Autodesk Inventor part; units mm, degrees
ref_plane "YZ Plane" through (0, 0, 0) normal (1, 0, 0) x (0, 1, 0)
ref_plane "XZ Plane" through (0, 0, 0) normal (0, 1, 0) x (-1, 0, 0)
ref_plane "XY Plane" through (0, 0, 0) normal (0, 0, 1) x (1, 0, 0)
sketch "Sketch1" plane through (0, 0, 0) normal (0, 1, 0) x (-1, 0, 0)
  line L0 (0, 0) -> (101.6, 0)
  line L1 (101.6, 0) -> (101.6, -101.6)
  line L2 (101.6, -101.6) -> (0, -101.6)
  line L3 (0, -101.6) -> (0, 0)
  dimension "d0" = 101.6
  dimension "d1" = 101.6
extrude "Extrusion1" add sketch "Sketch1" along normal blind 6.35 draft 0.25
sketch "Sketch2" plane through (0, 6.35, 0) normal (0, 1, 0) x (1, 0, 0)
  line L0 (-82.5492, 50.8025) -> (-86.8726, 48.5826)
  line L1 (-86.8726, 48.5826) -> (-82.3808, 47.537)
  line L2 (-82.3808, 47.537) -> (-86.5353, 45.4037)
  line L3 (-86.5353, 45.4037) -> (-81.9297, 44.5615)
  line L4 (-81.9297, 44.5615) -> (-85.8551, 42.0104)
  line L5 (-85.8551, 42.0104) -> (-81.2075, 41.6704)
  line L6 (-81.2075, 41.6704) -> (-84.931, 38.9182)
  line L7 (-84.931, 38.9182) -> (-80.2411, 38.9182)
  line L8 (-80.2411, 38.9182) -> (-83.7111, 35.8686)
  line L9 (-83.7111, 35.8686) -> (-78.9909, 36.1982)
  line L10 (-78.9909, 36.1982) -> (-82.2207, 32.9446)
  line L11 (-82.2207, 32.9446) -> (-77.3914, 33.4556)
  line L12 (-77.3914, 33.4556) -> (-80.2618, 29.8701)
  line L13 (-80.2618, 29.8701) -> (-75.5543, 30.9218)
  line L14 (-75.5543, 30.9218) -> (-78.0086, 27.0147)
  line L15 (-78.0086, 27.0147) -> (-73.2491, 28.3512)
  line L16 (-75.4686, 24.3897) -> (-70.7203, 26.0798)
  line L17 (-70.7203, 26.0798) -> (-72.3407, 21.7822)
  line L18 (-72.3407, 21.7822) -> (-67.7356, 23.947)
  line L19 (-67.7356, 23.947) -> (-68.5334, 19.3111)
  line L20 (-68.5334, 19.3111) -> (-64.1946, 22.0167)
  line L21 (-64.1946, 22.0167) -> (-64.3717, 17.3062)
  line L22 (-64.3717, 17.3062) -> (-60.4516, 20.5554)
  line L23 (-60.4516, 20.5554) -> (-60.1774, 15.8989)
  line L24 (-60.1774, 15.8989) -> (-56.5068, 19.5698)
  line L25 (-56.5068, 19.5698) -> (-55.1527, 14.9241)
  line L26 (-55.1527, 14.9241) -> (-52.5263, 19.0996)
  line L27 (-52.5263, 19.0996) -> (-50.7684, 14.6609)
  line L28 (-50.7684, 14.6609) -> (-48.585, 19.1298)
  line L29 (-48.585, 19.1298) -> (-46.5035, 14.9171)
  line L30 (-46.5035, 14.9171) -> (-45.1599, 19.5574)
  line L31 (-45.1599, 19.5574) -> (-42.5914, 15.6053)
  line L32 (-42.5914, 15.6053) -> (-41.7527, 20.3686)
  line L33 (-41.7527, 20.3686) -> (-39.298, 16.5397)
  line L34 (-39.298, 16.5397) -> (-38.6769, 21.4578)
  line L35 (-38.6769, 21.4578) -> (-35.49, 18.0635)
  line L36 (-35.49, 18.0635) -> (-35.1146, 23.1972)
  line L37 (-35.1146, 23.1972) -> (-30.9781, 20.581)
  line L38 (-30.9781, 20.581) -> (-31.5036, 25.5886)
  line L39 (-31.5036, 25.5886) -> (-27.2251, 23.4077)
  line L40 (-27.2251, 23.4077) -> (-28.4283, 28.2724)
  line L41 (-28.4283, 28.2724) -> (-23.9858, 26.5691)
  line L42 (-23.9858, 26.5691) -> (-26.0364, 30.9313)
  line L43 (-26.0364, 30.9313) -> (-21.3587, 29.8388)
  line L44 (-21.3587, 29.8388) -> (-23.7723, 34.1409)
  line L45 (-23.7723, 34.1409) -> (-18.848, 33.9105)
  line L46 (-18.848, 33.9105) -> (-22.0511, 37.3262)
  line L47 (-22.0511, 37.3262) -> (-17.264, 37.3262)
  line L48 (-17.264, 37.3262) -> (-20.7009, 40.6952)
  line L49 (-20.7009, 40.6952) -> (-15.918, 41.3408)
  line L50 (-15.918, 41.3408) -> (-19.7237, 44.293)
  line L51 (-19.7237, 44.293) -> (-15.0837, 45.2689)
  line L52 (-15.0837, 45.2689) -> (-19.1835, 47.8849)
  line L53 (-19.1835, 47.8849) -> (-14.7085, 48.8843)
  line L54 (-14.7085, 48.8843) -> (-19.0492, 50.8025)
  line L55 (-75.4686, 24.3897) -> (-73.2491, 28.3512)
  circle A0 centre (-50.8, 50.8) radius 31.7508
  circle A1 centre (-50.8, 50.8) radius 37.6285
  line L56 (-101.6277, 101.6277) -> (0.0277, 101.6277)
  line L57 (0.0277, 101.6277) -> (0.0277, -0.0277)
  line L58 (-101.6277, 101.6277) -> (0.0277, 101.6277)
  line L59 (0.0277, 101.6277) -> (0.0277, -0.0277)
  line L60 (0.0277, -0.0277) -> (-101.6277, -0.0277)
  line L61 (0.0277, -0.0277) -> (-101.6277, -0.0277)
  line L62 (-101.6277, -0.0277) -> (-101.6277, 101.6277)
extrude "Extrusion2" cut sketch "Sketch2" against normal blind 6.35 contours L56 L57 L60 L62
sketch "Sketch3" plane through (-50.8, 6.35, -50.8) normal (0, 1, 0) x (1, 0, 0)
  line L0 (-31.7492, 0.0025) -> (-36.0726, -2.2174)
  line L1 (-36.0726, -2.2174) -> (-31.5808, -3.263)
  line L2 (-31.5808, -3.263) -> (-35.7353, -5.3963)
  line L3 (-35.7353, -5.3963) -> (-31.1298, -6.2385)
  line L4 (-31.1298, -6.2385) -> (-35.0551, -8.7896)
  line L5 (-35.0551, -8.7896) -> (-30.4075, -9.1296)
  line L6 (-30.4075, -9.1296) -> (-34.131, -11.8818)
  line L7 (-34.131, -11.8818) -> (-29.4411, -11.8818)
  line L8 (-29.4411, -11.8818) -> (-32.9111, -14.9315)
  line L9 (-32.9111, -14.9315) -> (-28.191, -14.6019)
  line L10 (-28.191, -14.6019) -> (-31.4207, -17.8554)
  line L11 (-31.4207, -17.8554) -> (-26.5914, -17.3444)
  line L12 (-26.5914, -17.3444) -> (-29.4619, -20.9299)
  line L13 (-29.4619, -20.9299) -> (-24.7544, -19.8782)
  line L14 (-24.7544, -19.8782) -> (-27.2087, -23.7853)
  line L15 (-27.2087, -23.7853) -> (-22.4492, -22.4488)
  line L16 (-24.6686, -26.4103) -> (-19.9203, -24.7202)
  line L17 (-19.9203, -24.7202) -> (-21.5408, -29.0178)
  line L18 (-21.5408, -29.0178) -> (-16.9357, -26.853)
  line L19 (-16.9357, -26.853) -> (-17.7335, -31.489)
  line L20 (-17.7335, -31.489) -> (-13.3947, -28.7833)
  line L21 (-13.3947, -28.7833) -> (-13.5717, -33.4938)
  line L22 (-13.5717, -33.4938) -> (-9.6516, -30.2447)
  line L23 (-9.6516, -30.2447) -> (-9.3774, -34.9011)
  line L24 (-9.3774, -34.9011) -> (-5.7069, -31.2302)
  line L25 (-5.7069, -31.2302) -> (-4.3528, -35.8759)
  line L26 (-4.3528, -35.8759) -> (-1.7263, -31.7005)
  line L27 (-1.7263, -31.7005) -> (0.0315, -36.1391)
  line L28 (0.0315, -36.1391) -> (2.215, -31.6702)
  line L29 (2.215, -31.6702) -> (4.2964, -35.8829)
  line L30 (4.2964, -35.8829) -> (5.64, -31.2426)
  line L31 (5.64, -31.2426) -> (8.2086, -35.1948)
  line L32 (8.2086, -35.1948) -> (9.0473, -30.4314)
  line L33 (9.0473, -30.4314) -> (11.502, -34.2603)
  line L34 (11.502, -34.2603) -> (12.123, -29.3422)
  line L35 (12.123, -29.3422) -> (15.3099, -32.7365)
  line L36 (15.3099, -32.7365) -> (15.6854, -27.6028)
  line L37 (15.6854, -27.6028) -> (19.8219, -30.219)
  line L38 (19.8219, -30.219) -> (19.2964, -25.2114)
  line L39 (19.2964, -25.2114) -> (23.5749, -27.3924)
  line L40 (23.5749, -27.3924) -> (22.3717, -22.5276)
  line L41 (22.3717, -22.5276) -> (26.8141, -24.2309)
  line L42 (26.8141, -24.2309) -> (24.7636, -19.8687)
  line L43 (24.7636, -19.8687) -> (29.4412, -20.9612)
  line L44 (29.4412, -20.9612) -> (27.0277, -16.6591)
  line L45 (27.0277, -16.6591) -> (31.9519, -16.8895)
  line L46 (31.9519, -16.8895) -> (28.7489, -13.4738)
  line L47 (28.7489, -13.4738) -> (33.5359, -13.4738)
  line L48 (33.5359, -13.4738) -> (30.099, -10.1049)
  line L49 (30.099, -10.1049) -> (34.8819, -9.4592)
  line L50 (34.8819, -9.4592) -> (31.0763, -6.5071)
  line L51 (31.0763, -6.5071) -> (35.7163, -5.5311)
  line L52 (35.7163, -5.5311) -> (31.6164, -2.9151)
  line L53 (31.6164, -2.9151) -> (36.0915, -1.9157)
  line L54 (36.0915, -1.9157) -> (31.7508, 0.0025)
  line L55 (-24.6686, -26.4103) -> (-22.4492, -22.4488)
  line L56 (-31.7492, 0.0025) -> (31.7508, 0.0025)
  circle A0 centre (0.0008, 0.0025) radius 37.6862
  point P0 (50.8, -50.8)
extrude "Extrusion3" cut sketch "Sketch3" against normal blind 6.35
For this review, take the finished solid that the model builds, in its own axes (mm). A direction names the side the tool comes from. Coordinates: 2 decimals unless noted, no trailing zeros. Write each loop counter-clockwise with the first axis right and the second up, starting at its lowest first coordinate (ties: lowest second). Pieces come first, ordered by that corner, then holes.
(1) Tool access review of faces 1 (the face through (-27.82, 3.22, -25.81)), 2 (the face through (-51.66, 3.22, -16.91)), 3 (the face through (-16.85, 3.22, -49.83)), 4 (the face through (-18.343, 3.219, -41.013)): name each direction out of +Z, -Z, +X, -X, +Y, -Y from which nothing blocks a thin tool from reaching the whole face with its end or side.
(2) Wall thickness on probe 1 along X at (y, z) = (0.5, -21); probe 2 along Z at (x, y) = (-80.5, 3.75); probe 3 along Z at (x, y) = (-23.5, 1.5): over which ranges is each line inside the solid? List them lowest first.
(3) The part is to be moulded in two halves that separate along X. For faces 5 (the face through (-81.38, 3.22, -36.03)), 6 (the face through (-17.8, 3.2, -42.8)), 7 (the face through (-58.368, 3.219, -17.709)), say which applies: +X half, -X half, draft (parallel to the pull), parting line (faces both ways), or undercut.
(4) For pin 1 Ø1 at (y, z) = (4.5, -24) entering from -X; pin 2 Ø1 at (y, z) = (1, -25) entering from +X; pin 3 Ø1 at (y, z) = (0.5, -29) entering from +X, all flat-tipped, find the tip position at first contact; note any pin that passes through.
(5) Add section B-B on x = -43.5. Give the boundary of the cut face in (y, z), then the cut area to 3 significant figures.
(6) Add section C-C on z = -43.5. Give the boundary of the cut face in (x, y), then the cut area to 3 significant figures.
(7) Add section A-A on x = -74. Give the boundary of the cut face in (y, z), then the cut area to 3 significant figures.
Answer sheet:
1. face 1: +Y, -Y
1. face 2: +Z, +Y, -Y
1. face 3: -Z, +X, +Y, -Y
1. face 4: +X, +Y, -Y
2. probe 1: x = -68.24 to -65.83, -64.23 to -38.73, -38.25 to -35.28, -31.64 to -31.02
2. probe 2: z = -50.8 to -38.92, -38.69 to -36.09, -34.68 to -33.13
2. probe 3: z = -50.8 to -34.13, -33.66 to -30.34
3. face 5: undercut
3. face 6: +X half
3. face 7: undercut
4. pin 1: stops at x = -75.47
4. pin 2: stops at x = -27.5
4. pin 3: stops at x = -24.89
5. outline: (0, -50.8) - (6.35, -50.8) - (6.35, -17) - (0, -17) - close
5. area: 215 mm2
6. outline: (-83.56, 0) - (-18.7, 0) - (-18.7, 6.35) - (-83.56, 6.35) - close
6. area: 412 mm2
7. outline: (0, -50.8) - (6.35, -50.8) - (6.35, -28.14) - (0, -28.14) - close; (0, -27.01) - (6.35, -27.01) - (6.35, -24.91) - (0, -24.91) - close
7. area: 157 mm2
